Input: dimensioned drawing with shaded views. Units: mm. Origin: part minimum x, y, z. A direction names the side the tool comes from. Give positions to 0.01 mm unless a question says otherwise; leave off trailing zeros. Loops run counter-clockwise (first coordinate to the right, second up) from the corner with the lowest first, then second, coordinate; pieces in that order, holes last. Notation, with made-up numbers: (69, -3.75) -> (107, -3.75) arc R25 cw to (107, 13.25) -> close; hole circle Ø10 at (21.25, -22). An arc over 180 degrees is marked (long way). Answer as a JSON object with one key per item and string values.
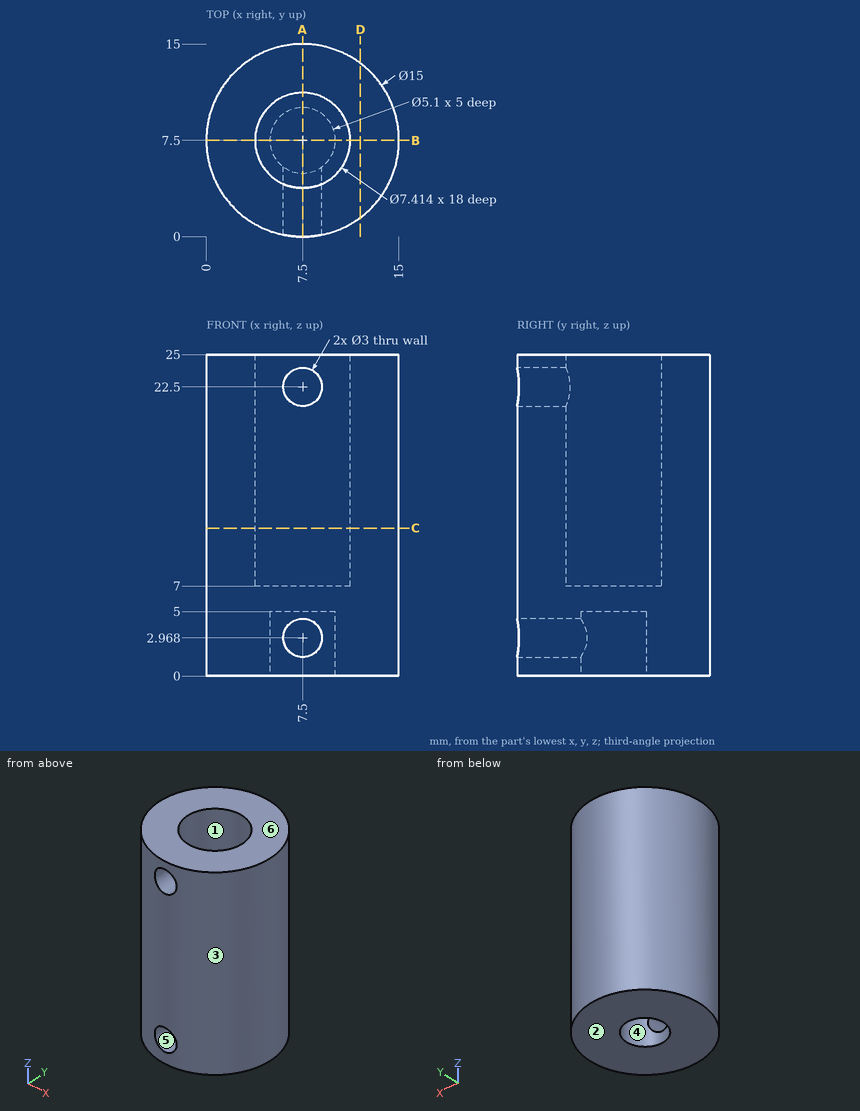
Q1. Pin query (flat end, axial travel): pin 1 (5 mm diameter, centred on x = 7, z = 5.5, fed in from -Y); pin 2 (6 mm diameter, centred on x = 12.5, z = 6.5, fed in from +Y); pin 3 (1.5 mm diameter, centred on y = 13.5, z = 8, fed in from -X) (1 decimal); pin 4 (4.5 mm diameter, centred on x = 7.5, y = 7.5, fed in from -Z). Return the tip coordinate at first contact, or that it passes through.
Evaluation:
{"pin 1": "stops at y = 0", "pin 2": "stops at y = 14.73", "pin 3": "stops at x = 2.1", "pin 4": "stops at z = 5"}
Q2. Section B-B, the plane y = 7.5. Return the cut outline in (x, z), then the cut area to 3 significant figures.
Evaluation:
{"outline": "(0, 0) -> (4.95, 0) -> (4.95, 5) -> (10.05, 5) -> (10.05, 0) -> (15, 0) -> (15, 25) -> (11.21, 25) -> (11.21, 7) -> (3.79, 7) -> (3.79, 25) -> (0, 25) -> close", "area": "216 mm2"}
Q3. Section A-A, the plane x = 7.5. Return the cut outline in (y, z).
Evaluation:
{"outline": "(0, 0) -> (4.95, 0) -> (4.95, 1.47) -> (0, 1.47) -> close; (0, 4.47) -> (4.95, 4.47) -> (4.95, 5) -> (10.05, 5) -> (10.05, 0) -> (15, 0) -> (15, 25) -> (11.21, 25) -> (11.21, 7) -> (3.79, 7) -> (3.79, 21) -> (0, 21) -> close; (0, 24) -> (3.79, 24) -> (3.79, 25) -> (0, 25) -> close"}
Q4. Draft query along X for the marked faces 1, 2 and 3. Return one class per face: +X half, -X half, draft (parallel to the pull), parting line (faces both ways), or undercut.
Evaluation:
{"face 1": "undercut", "face 2": "draft", "face 3": "parting line"}
Q5. Section D-D, the plane x = 12. Return the cut outline in (y, z), then the cut area to 3 significant figures.
Evaluation:
{"outline": "(1.5, 0) -> (13.5, 0) -> (13.5, 25) -> (1.5, 25) -> close", "area": "300 mm2"}
Q6. Ray query, line 1 along Y through (x, z) = (7.5, 19); line 2 along X through (y, z) = (5.75, 7.5); line 3 along Y through (x, z) = (7.5, 1.5). Return the intervals inside material, ascending.
Evaluation:
{"line 1": "y = 0 to 3.79, 11.21 to 15", "line 2": "x = 0.21 to 4.23, 10.77 to 14.79", "line 3": "y = 10.05 to 15"}
Q7. Access query for the marked faces 4, 5 and 6. Directions: +Z, -Z, +X, -X, +Y, -Y. A direction counts if a zero-diameter tool reaches every point of the face in a straight line with its end or side. Return the directions, or none.
Evaluation:
{"face 4": "-Z", "face 5": "-Y", "face 6": "+Z, +X, -X, +Y, -Y"}
Q8. Section C-C, the plane z = 11.5. Return the cut outline in (x, y).
Evaluation:
{"outline": "circle Ø15 at (7.5, 7.5); hole circle Ø7.41 at (7.5, 7.5)"}
